Input: part model. Units: mm. Frame: model coordinates. Coordinates: 2 decimals unless noted, no trailing zeros. Loops run counter-clockwise (first coordinate to the right, second up) from the corner with the lowest first, then second, coordinate; pieces in that order, holes last. Notation, with made-up numbers: (-33.75, 76) - (-0.75, 76) arc R30 cw to (-0.75, 113) - close; hole circle Ø3 at (-23, 85). An arc over 180 degrees is marked (long way). Answer as CSV lines item,"result". Start each with the question number.
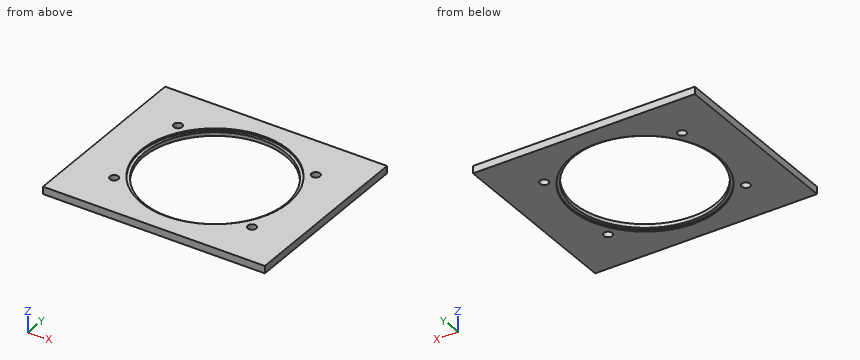
```python
from build123d import *

# Parameters (mm, degrees)
F0_W     = 600
F0_H     = 500
F0_R     = 192
F1_DEPTH = 20
F2_R     = 11.5
F3_DEPTH = 20
F4_R     = 200
F5_DEPTH = 5
F6_R     = 200
F7_DEPTH = 5


with BuildPart() as f1:
    # F0 (on Top) → F1 (new body)
    with BuildSketch(Plane.XY):
        Rectangle(F0_W, F0_H)
        Circle(F0_R, mode=Mode.SUBTRACT)
    extrude(amount=F1_DEPTH)

    # F2 (on face) → F3 (cut, through all)
    with BuildSketch(Plane.XY.offset(20)):
        with Locations((186.35709, 130.488639)):
            Circle(F2_R)
        with Locations((-186.35709, 130.488639)):
            Circle(F2_R)
        with Locations((-186.35709, -130.488639)):
            Circle(F2_R)
        with Locations((186.35709, -130.488639)):
            Circle(F2_R)
    extrude(amount=-F3_DEPTH, mode=Mode.SUBTRACT)

    # F4 (on face) → F5 (cut)
    with BuildSketch(Plane(origin=(0, 0, 0), x_dir=(1, 0, 0), z_dir=(0, 0, -1))):
        Circle(F4_R)
    extrude(amount=-F5_DEPTH, mode=Mode.SUBTRACT)

    # F6 (on face) → F7 (cut)
    with BuildSketch(Plane.XY.offset(20)):
        Circle(F6_R)
    extrude(amount=-F7_DEPTH, mode=Mode.SUBTRACT)


solid = f1.part
```
Item 1: Section query B-B, the plane y = 0. Output: boundary loops of the cut face in (x, z), and give its area (3 significant figures).
Item 2: Section query A-A, the plane x = 0. Output: boundary loops of the cut face in (y, z).
Item 3: Section query C-C, the plane z = 9. Output: boundary loops of the cut face in (x, y), and give its area (3 significant figures).
Item 4: Contact query for a flat-ended pin moving along its axis: P1, Ø18.5, axis at x = 186.36, y = 130.49, coming from the -Z side. Output: stop coordinate, or through.
Item 5: Material intervals for probe 1 along Y at (x, z) = (3, 1.25); probe 2 along X at (y, z) = (0, 7); probe 3 along Y at (x, z) = (-6, 7.75), sorted ascending.
Response values:
1,outline,"(-300, 0) - (-200, 0) - (-200, 5) - (-192, 5) - (-192, 15) - (-200, 15) - (-200, 20) - (-300, 20) - close; (192, 5) - (200, 5) - (200, 0) - (300, 0) - (300, 20) - (200, 20) - (200, 15) - (192, 15) - close"
1,area,"4,160 mm²"
2,outline,"(-250, 0) - (-200, 0) - (-200, 5) - (-192, 5) - (-192, 15) - (-200, 15) - (-200, 20) - (-250, 20) - close; (192, 5) - (200, 5) - (200, 0) - (250, 0) - (250, 20) - (200, 20) - (200, 15) - (192, 15) - close"
3,outline,"(-300, -250) - (300, -250) - (300, 250) - (-300, 250) - close; hole circle Ø23 at (-186.36, -130.49); hole circle Ø23 at (-186.36, 130.49); hole circle Ø384 at (0, 0); hole circle Ø23 at (186.36, -130.49); hole circle Ø23 at (186.36, 130.49)"
3,area,"183,000 mm²"
4,P1,"passes through"
5,probe 1,"y = -250 to -199.98, 199.98 to 250"
5,probe 2,"x = -300 to -192, 192 to 300"
5,probe 3,"y = -250 to -191.91, 191.91 to 250"
